Source: three-view drawing plus pictorial views. Frame: mm from the lowest corner of the part. Give positions to 0.01 mm unless a question says otherwise; leave off trailing zeros. Order: outer loops, then holes, each group sorted by start corner. A loop starts at its lowest first (then second) coordinate and runs counter-clockwise, first axis right, second up. Notation, with made-up numbers: (46.5, 71.25) -> (79.5, 71.25) arc R9 ccw to (79.5, 85.25) -> close; hole circle Ø7 at (-21, -4.75). An arc over 180 degrees is marked (long way). Write item = value, one per line.
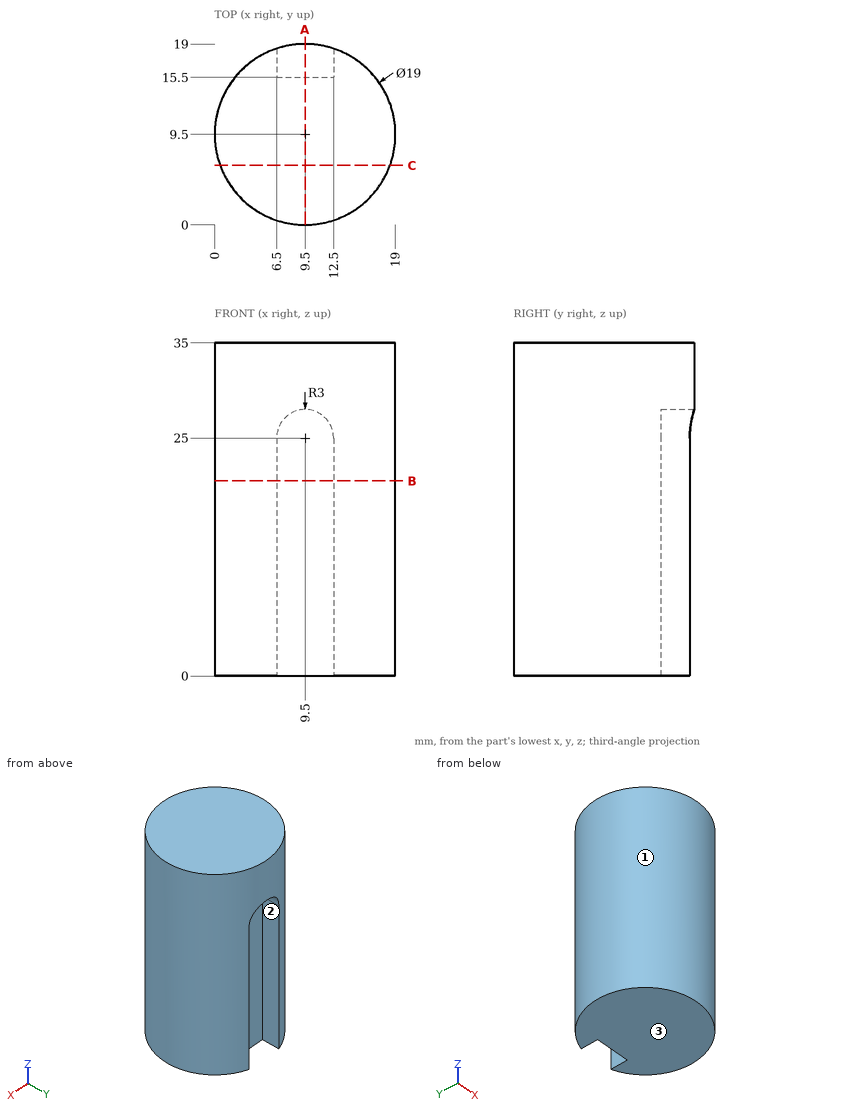
1) Section query C-C (y = 6.25). Output: boundary loops of the cut face in (x, z), plus the area to 3 significant figures.
Check sheet entries:
outline = (0.57, 0) -> (18.43, 0) -> (18.43, 35) -> (0.57, 35) -> close
area = 625 mm²
2) Section query B-B (z = 20.5). Output: boundary loops of the cut face in (x, y).
Check sheet entries:
outline = (6.5, 15.5) -> (6.5, 18.51) arc R9.5 ccw (long way) to (12.5, 18.51) -> (12.5, 15.5) -> close
3) Section query A-A (x = 9.5). Output: boundary loops of the cut face in (y, z), plus the area to 3 significant figures.
Check sheet entries:
outline = (0, 0) -> (15.5, 0) -> (15.5, 28) -> (19, 28) -> (19, 35) -> (0, 35) -> close
area = 567 mm²
4) Line query: line 1 (X direction, y = 17.5, z = 17); line 2 (X direction, y = 16.5, z = 17); line 3 (Y direction, x = 8.25, z = 26.5). Output: solid intervals per line, ascending. Write a range as from..to.
Check sheet entries:
line_1 = 4.38..6.5, 12.5..14.62
line_2 = 3.08..6.5, 12.5..15.92
line_3 = 0.08..15.5
5) Mould query, pull axis X, two halves, no side actions, for the marked faces 1, 2 and 3. Classes: +X half, -X half, draft (parallel to the pull), parting line (faces both ways), or undercut.
Check sheet entries:
face_1 = parting line
face_2 = undercut
face_3 = draft
6) First-contact query: P1, Ø6.5, axis at x = 8.5, z = 12, coming from the +Y side; P2, Ø1.5, axis at y = 16.5, z = 11, coming from the -X side; P3, Ø10, axis at y = 3, z = 21, coming from the -X side. Flat tips, straight axial feed; report the tip coordinate or a pass-through.
Check sheet entries:
P1 = 18.51
P2 = 2.35
P3 = 0.12
